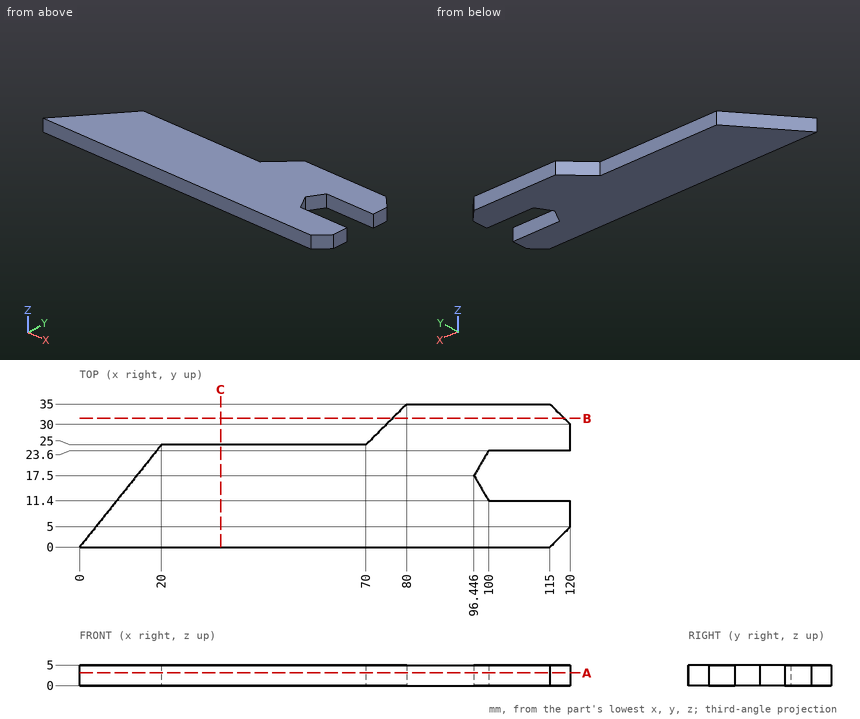
Could you check a few things on this drawing? It's one solid part, dimensions in mm from its lowest x, y, z. Round coordinates to 2 decimals unless told otherwise and drop trailing zeros. Order: outer loops, then holes, each group sorted by start corner. A loop starts at its lowest first (then second) coordinate and runs counter-clockwise, first axis right, second up. Notation, with made-up numbers: M 49.25,58.25 L 64.25,58.25 A11 ccw 64.25,62.25 Z; hole C -17.75,72.25 d6. An arc over 180 degrees is marked long. One line per question, with ' | ' between items.
1) Imagine slicing it at B-B, the plane y = 31.5. Write out the boundary of the cut face in (x, z), plus the area to 3 significant figures.
Checked values:
outline: M 76.5,0 L 118.5,0 L 118.5,5 L 76.5,5 Z | area: 210 mm²
2) Imagine slicing it at A-A, the plane z = 3.1. Write out the boundary of the cut face in (x, y) (1 decimal).
Checked values:
outline: M 0,0 L 115,0 L 120,5 L 120,11.4 L 100,11.4 L 96.4,17.5 L 100,23.6 L 120,23.6 L 120,30 L 115,35 L 80,35 L 70,25 L 20,25 Z
3) Imagine slicing it at C-C, the plane x = 34.5. Write out the boundary of the cut face in (y, z).
Checked values:
outline: M 0,0 L 25,0 L 25,5 L 0,5 Z
4) I'm going to push flat-ended pins straight in: pin 1 Ø2 at (x, z) = (57, 1) entering from +Y; pin 2 Ø1 at (y, z) = (19.5, 2) entering from +X. Where does each tip first touch, or does it pass through?
Checked values:
pin 1: stops at y = 25 | pin 2: stops at x = 97.9
5) I need wall thicknesses on line 1 (Y direction, x = 106.5, z = 0.3); line 2 (Y direction, x = 36, z = 3.6); line 3 (X direction, y = 21, z = 3.35) (1 decimal). Which ranges of each line are inside material? Lowest first, please.
Checked values:
line 1: y = 0 to 11.4, 23.6 to 35 | line 2: y = 0 to 25 | line 3: x = 16.8 to 98.5
